Source: CAD feature listing. Evaluate the final solid. Frame: model axes, mm. Face numbers are marked on the shaded views. A direction names the side the tool comes from. Round coordinates to 2 decimals unless told otherwise and drop trailing zeros. Order: outer loops, then holes, each group sorted by start corner. A loop starts at its lowest first (then second) coordinate and runs counter-clockwise, first axis right, second up. Notation, with made-up numbers: (3, -18) -> (7, -18) arc R18 cw to (7, -9) -> close; hole circle Ø7 at (49.5, 84.25). An arc over 180 degrees is marked (long way). Answer as CSV lines item,"result".
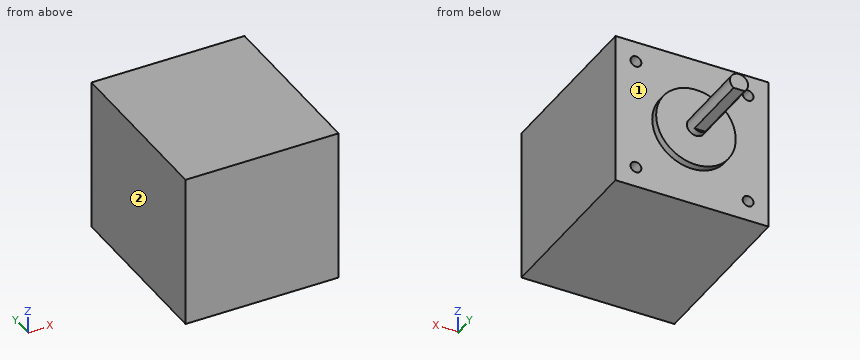
from build123d import *

# Parameters (mm, degrees)
SKETCH1_W           = 42.3
SKETCH1_H           = 42.3
BOSS_EXTRUDE1_DEPTH = 48
SKETCH2_R           = 11
BOSS_EXTRUDE2_DEPTH = 2
SKETCH3_R           = 2.5
BOSS_EXTRUDE3_DEPTH = 24
SKETCH4_R           = 1.5
CUT_EXTRUDE1_DEPTH  = 4
CUT_EXTRUDE2_DEPTH  = 20


with BuildPart() as part:
    # Sketch1 → Boss-Extrude1 (new body)
    with BuildSketch(Plane(origin=(0, 0, 0), x_dir=(1, 0, 0), z_dir=(0, 1, 0))):
        Rectangle(SKETCH1_W, SKETCH1_H)
    extrude(amount=BOSS_EXTRUDE1_DEPTH)

    # Sketch2 → Boss-Extrude2 (add)
    with BuildSketch(Plane(origin=(0, 48, 0), x_dir=(1, 0, 0), z_dir=(0, 1, 0))):
        Circle(SKETCH2_R)
    extrude(amount=BOSS_EXTRUDE2_DEPTH)

    # Sketch3 → Boss-Extrude3 (add)
    with BuildSketch(Plane(origin=(0, 48, 0), x_dir=(1, 0, 0), z_dir=(0, 1, 0))):
        Circle(SKETCH3_R)
    extrude(amount=BOSS_EXTRUDE3_DEPTH)

    # Sketch4 → Cut-Extrude1 (cut)
    with BuildSketch(Plane(origin=(0, 48, 0), x_dir=(1, 0, 0), z_dir=(0, 1, 0))):
        with Locations((15.5, 15.5)):
            Circle(SKETCH4_R)
        with Locations((15.5, -15.5)):
            Circle(SKETCH4_R)
        with Locations((-15.5, 15.5)):
            Circle(SKETCH4_R)
        with Locations((-15.5, -15.5)):
            Circle(SKETCH4_R)
    extrude(amount=-CUT_EXTRUDE1_DEPTH, mode=Mode.SUBTRACT)

    # Sketch5 → Cut-Extrude2 (cut)
    with BuildSketch(Plane(origin=(0, 72, 0), x_dir=(1, 0, 0), z_dir=(0, 1, 0))):
        Polygon((-76.274840795, 2), (-1.5, 2), (1.5, 2), (76.274840795, 2), (76.274840795, 151.54968159), (-76.274840795, 151.54968159), align=None)
    extrude(amount=-CUT_EXTRUDE2_DEPTH, mode=Mode.SUBTRACT)


solid = part.part
1. Section query D-D on x = -15.5. Return loops of the section in (y, z), and give its area (3 significant figures).
Results below:
outline,"(0, -21.15) -> (48, -21.15) -> (48, -17) -> (44, -17) -> (44, -14) -> (48, -14) -> (48, 14) -> (44, 14) -> (44, 17) -> (48, 17) -> (48, 21.15) -> (0, 21.15) -> close"
area,"2,010 mm2"
2. Section query B-B on x = 0. Return loops of the section in (y, z), and give its area (3 significant figures).
Results below:
outline,"(0, -21.15) -> (48, -21.15) -> (48, -11) -> (50, -11) -> (50, -2.5) -> (52, -2.5) -> (52, -2) -> (72, -2) -> (72, 2.5) -> (50, 2.5) -> (50, 11) -> (48, 11) -> (48, 21.15) -> (0, 21.15) -> close"
area,"2,170 mm2"
3. Pin query (flat end, axial travel): pin 1 (1.5 mm diameter, centred on x = -16, z = 15.5, fed in from +Y); pin 2 (12 mm diameter, centred on x = -10.5, z = -8.5, fed in from +Y); pin 3 (4 mm diameter, centred on x = -15.5, z = -15.5, fed in from +Y). Return the tip coordinate at first contact, or that it passes through.
Results below:
pin 1,"y = 44"
pin 2,"y = 50"
pin 3,"y = 48"
4. Line query: L1, parallel to X at y = 45.25, z = 15.5; L2, parallel to Z at x = -15, y = 45. Output: solid intervals per line, ascending. Write a range as [from, to].
Results below:
L1,"[-21.15, -17], [-14, 14], [17, 21.15]"
L2,"[-21.15, -16.91], [-14.09, 14.09], [16.91, 21.15]"
5. Reachability of the marked faces 1 and 2 from +Z, -Z, +X, -X, +Y, -Y: full face, straight path, thin tool, end or side. Return the list, or none.
Results below:
face 1,"+Y"
face 2,"+Z, -Z, -X, +Y, -Y"
6. Section query A-A on z = 0. Return loops of the section in (x, y).
Results below:
outline,"(-21.15, 0) -> (21.15, 0) -> (21.15, 48) -> (11, 48) -> (11, 50) -> (2.5, 50) -> (2.5, 72) -> (-2.5, 72) -> (-2.5, 50) -> (-11, 50) -> (-11, 48) -> (-21.15, 48) -> close"
7. Section query C-C on y = 56.5. Return loops of the section in (x, z).
Results below:
outline,"(-1.5, -2) -> (1.5, -2) arc R2.5 ccw (long way) to start"
